Could you check a few things on this model? Use its own coordinates, in mm. Give positions to 0.01 mm unless a question says otherwise; leave off trailing zeros. Loops run counter-clockwise (first coordinate to the right, second up) from the corner with the lowest first, then second, coordinate; pieces in that order, holes last. Notation, with made-up numbers: M -4,52.25 L 39,52.25 A24 ccw 39,76.25 Z; hole C 28.5,23.5 d2. An arc over 180 degrees is marked long. Use a Markdown table: item, result. Add a question column.
1) If I drill on line 1 along Z through (x, y) = (-122.5, -5.75); line 2 along Z through (x, y) = (-132.5, 2.5); line 3 along X through (y, z) = (0.25, 15), over which ranges is the centre line in solid material (lowest first)? Write a range as [from, to].
2) Suppose I cut it at A-A on z = 35. List the corners of the cut face in (x, y) for me (3 decimals).
3) Suppose I cut it at B-B on x = 126.5. Count the separate pieces of the cut face and the enclosed holes in it, and give its area (3 significant figures).
4) Will these pins go through, and if not, where does the flat tip stop? pin 1 Ø1.6 at (x, y) = (-200, 2) entering from -Z; pin 2 Ø1.9 at (x, y) = (-199, -4) entering from +Z; pin 3 Ø1.6 at (y, z) = (1, 14) entering from -X.
5) Suppose I cut it at C-C on y = -3. List the corners of the cut face in (x, z) for me, and give its area (3 significant figures).
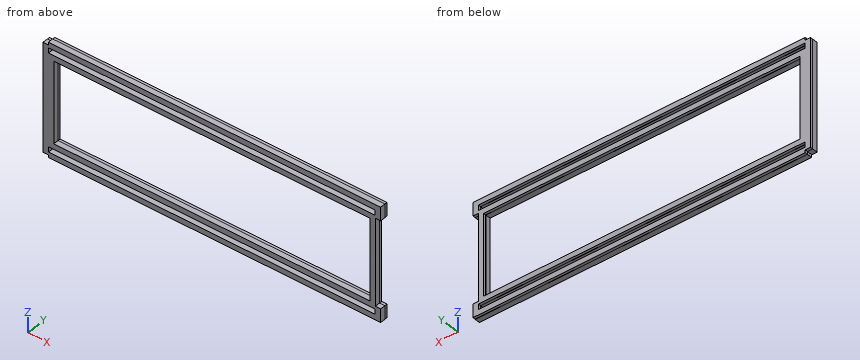
```python
from build123d import *

# Parameters (mm, degrees)
SKETCH1_W           = 393.6492
SKETCH1_H           = 6.4008
SKETCH1_W_2         = 380.8984
SKETCH1_H_2         = 97.44075
BOSS_EXTRUDE1_DEPTH = 3.175
SKETCH5_W           = 393.446
SKETCH5_H           = 6.1976
SKETCH5_W_2         = 380.6952
SKETCH5_H_2         = 97.23755
BOSS_EXTRUDE4_DEPTH = 6.35


with BuildPart() as part:
    # Sketch1 → Boss-Extrude1 (new body)
    with BuildSketch(Plane(origin=(0, 0, 0), x_dir=(1, 0, 0), z_dir=(0, 1, 0))):
        Polygon((-203.2, 64.620775), (-203.2, -64.620775), (-196.85, -64.620775), (-196.85, -67.821175), (203.2, -67.821175), (203.2, -51.895375), (196.7992, -51.895375), (196.7992, 51.895375), (203.2, 51.895375), (203.2, 67.821175), (-196.85, 67.821175), (-196.85, 64.620775), align=None)
        with Locations((-0.0254, 58.270775)):
            Rectangle(SKETCH1_W, SKETCH1_H, mode=Mode.SUBTRACT)
        with Locations((-0.0254, -58.270775)):
            Rectangle(SKETCH1_W, SKETCH1_H, mode=Mode.SUBTRACT)
        Rectangle(SKETCH1_W_2, SKETCH1_H_2, mode=Mode.SUBTRACT)
    extrude(amount=BOSS_EXTRUDE1_DEPTH)

    # Sketch5 → Boss-Extrude4 (add)
    with BuildSketch(Plane(origin=(0, 0, 0), x_dir=(-1, 0, 0), z_dir=(0, -1, 0))):
        Polygon((-203.3016, -51.793775), (-203.3016, -67.922775), (196.9516, -67.922775), (196.9516, -64.722375), (203.3016, -64.722375), (203.3016, 64.722375), (196.9516, 64.722375), (196.9516, 67.922775), (-203.3016, 67.922775), (-203.3016, 51.793775), (-196.9008, 51.793775), (-196.9008, -51.793775), align=None)
        with Locations((0.0254, 58.270775)):
            Rectangle(SKETCH5_W, SKETCH5_H, mode=Mode.SUBTRACT)
        Rectangle(SKETCH5_W_2, SKETCH5_H_2, mode=Mode.SUBTRACT)
        with Locations((0.0254, -58.270775)):
            Rectangle(SKETCH5_W, SKETCH5_H, mode=Mode.SUBTRACT)
    extrude(amount=BOSS_EXTRUDE4_DEPTH)


solid = part.part
```
Answer block:
| question | item | result |
|---|---|---|
| 1 | line 1 | z = [-67.92, -61.37], [-55.17, -48.62], [48.62, 55.17], [61.37, 67.92] |
| 1 | line 2 | z = [-67.82, -61.47], [-55.07, -48.72], [48.72, 55.07], [61.47, 67.82] |
| 1 | line 3 | x = [-203.2, -190.45], [190.45, 196.8] |
| 2 | outline | M -203.302,-6.35 L -190.348,-6.35 L -190.348,0 L -190.449,0 L -190.449,3.175 L -203.2,3.175 L -203.2,0 L -203.302,0 Z; M 190.348,-6.35 L 196.901,-6.35 L 196.901,0 L 196.799,0 L 196.799,3.175 L 190.449,3.175 L 190.449,0 L 190.348,0 Z |
| 3 | separate pieces | 4 |
| 3 | enclosed holes | 0 |
| 3 | area | 247 mm^2 |
| 4 | pin 1 | stops at z = -64.62 |
| 4 | pin 2 | stops at z = 64.72 |
| 4 | pin 3 | stops at x = -203.2 |
| 5 | outline | M -203.3,-64.72 L -196.95,-64.72 L -196.95,-67.92 L 203.3,-67.92 L 203.3,-51.79 L 196.9,-51.79 L 196.9,51.79 L 203.3,51.79 L 203.3,67.92 L -196.95,67.92 L -196.95,64.72 L -203.3,64.72 Z; hole M -196.75,-61.37 L 196.7,-61.37 L 196.7,-55.17 L -196.75,-55.17 Z; hole M -196.75,55.17 L 196.7,55.17 L 196.7,61.37 L -196.75,61.37 Z; hole M -190.35,-48.62 L 190.35,-48.62 L 190.35,48.62 L -190.35,48.62 Z |
| 5 | area | 12,600 mm^2 |
